Design review of the part built by this model. Coordinates are the model's own, in mm. A direction names the side the tool comes from. Give positions to 0.01 mm unless a question says otherwise; leave off trailing zeros. Use one line per item in the form item = value. Start each with the question number.
from build123d import *

# Parameters (mm, degrees)
EXTRUDE_THIN1_DEPTH = 555.625
FILLET1_R           = 1.27


with BuildPart() as part:
    # Sketch1 → Extrude-Thin1 (new body)
    with BuildSketch(Plane.XY):
        with BuildLine():
            Line((0, 0), (0, -11.1125))
            Line((0, -11.1125), (-9.525, -11.1125))
            Line((-9.525, -11.1125), (-9.525, -4.7625))
            ThreePointArc((-9.525, -4.7625), (-15.689105931, -2.896158896), (-19.782692308, 2.075961538))
            Line((-19.782692308, 2.075961538), (-24.667307692, 13.799038462))
            ThreePointArc((-24.667307692, 13.799038462), (-28.760894069, 18.771158896), (-34.925, 20.6375))
            Line((-34.925, 20.6375), (-34.925, 44.45))
            Line((-34.925, 44.45), (-22.225, 44.45))
            Line((-22.225, 44.45), (-22.225, 43.18))
            Line((-22.225, 43.18), (-33.655, 43.18))
            Line((-33.655, 43.18), (-33.655, 21.842199611))
            ThreePointArc((-33.655, 21.842199611), (-27.536436435, 19.46157057), (-23.495, 14.2875))
            Line((-23.495, 14.2875), (-18.610384615, 2.564423077))
            ThreePointArc((-18.610384615, 2.564423077), (-14.443755021, -2.175295027), (-8.255, -3.410220605))
            Line((-8.255, -3.410220605), (-8.255, -9.8425))
            Line((-8.255, -9.8425), (-1.27, -9.8425))
            Line((-1.27, -9.8425), (-1.27, 0))
            Line((-1.27, 0), (0, 0))
        make_face()
    extrude(amount=-EXTRUDE_THIN1_DEPTH)

    # Fillet1
    fillet1_edges = [part.edges().sort_by_distance(p)[0] for p in [
        (-8.255, -3.410220605, -277.8125),
        (0, -11.1125, -277.8125),
        (-9.525, -11.1125, -277.8125),
        (-34.925, 20.6375, -277.8125),
        (-34.925, 44.45, -277.8125),
    ]]
    fillet(fillet1_edges, radius=FILLET1_R)


solid = part.part
1. To check wall thickness, follow L1, parallel to X at y = -8, z = -487.5 (3 decimals); L2, parallel to Y at x = -3, z = -358; L3, parallel to X at y = 32, z = -197 (3 decimals). State the ranges of each line that lie inside material, in increasing order.
2. Draft analysis for pull direction X (two halves, no side actions). For faces 4 (the flat face through (-1.27, -5, -274)), 5 (the flat face through (0, -5, -274)), 6 (the cylindrical face through (-28.227, 18.392, -273.923)), state which applies: pulls with the +X half, pulls with the -X half, needs draft (parallel to the pull), parting line crosses it, or undercut.
3. For faces 1 (the flat face through (-22.191, 7.855, -273.923)), 2 (the cylindrical face through (-15.052, -1.794, -273.923)), 3 (the flat face through (-28, 43.18, -274)), list the 3-axis set-ups (+Z, -Z, +X, -X, +Y, -Y) from which the entire face can be reached by the end or side of a thin tool; tool diameter is ignored.
4. Clearance check with flat-ended pins moving along their axes: pin 1 Ø10 at (y, z) = (10.5, -451) entering from -X; pin 2 Ø12 at (x, z) = (-25.5, -122) entering from -Y; pin 3 Ø17 at (y, z) = (36, -376) entering from +X (3 decimals). State where each tip first meets the part, or that it passes through.
Answer block:
q1.L1 = -9.525 to -8.255, -1.27 to 0
q1.L2 = -11.11 to -9.84
q1.L3 = -34.925 to -33.655
q2.face_4 = undercut
q2.face_5 = pulls with the +X half
q2.face_6 = pulls with the -X half
q3.face_1 = +Z, -Z, -X, -Y
q3.face_2 = +Z, -Z, +Y
q3.face_3 = +Z, -Z, +X
q4.pin_1 = -25.56
q4.pin_2 = 1.45
q4.pin_3 = -22.225
